Verification items for the finished model (mm, model axes). Face numbers are marked on the shaded views. A direction names the side the tool comes from. Give positions to 0.01 mm unless a question says otherwise; leave off trailing zeros. Loops run counter-clockwise (first coordinate to the right, second up) from the corner with the lowest first, then second, coordinate; pieces in that order, holes last. Notation, with made-up numbers: M 36.5,14.5 L 91.5,14.5 A33 ccw 91.5,46.5 Z; hole C -39,10 d4. An arc over 180 degrees is marked long. Answer in a Markdown table with one row per item.
```python
from build123d import *

# Parameters (mm, degrees)
ESBO_O1_W                        = 56
ESBO_O1_H                        = 28.051471863
RESSALTO_EXTRUS_O1_DEPTH         = 16
CORTE_EXTRUS_O1_DEPTH            = 100
ESBO_O3_W                        = 18
ESBO_O3_H                        = 28.051471863
CORTE_EXTRUS_O2_DEPTH            = 5
FURO_COM_FOLGA_DE_M32_D          = 3.4
FURO_COM_FOLGA_DE_M34_D          = 3.4
CHANFRO1_SIZE                    = 5
CORTE_EXTRUS_O3_DEPTH            = 8
RESSALTO_EXTRUS_O3_DEPTH         = 56
CORTE_EXTRUS_O4_DEPTH            = 100
CHANFRO2_START                   = 38.631741411
CHANFRO2_OUTLINE_W               = 9
CHANFRO2_OUTLINE_H               = 10
CHANFRO2_DEPTH                   = 4.368258589
CHANFRO3_START                   = -67
CHANFRO3_OUTLINE_W               = 9
CHANFRO3_OUTLINE_H               = 10
CHANFRO3_DEPTH                   = 3.439248526
RESSALTO_EXTRUS_O4_DEPTH         = 2
CORTE_EXTRUS_O5_DEPTH            = 100
CORTE_EXTRUS_O6_START            = -56
ESBO_O24_W                       = 1.5
ESBO_O24_H                       = 30.126471863
CORTE_EXTRUS_O6_DEPTH            = 56
RESSALTO_EXTRUS_O6_DEPTH         = 17
RESSALTO_EXTRUS_O7_START         = -17
RESSALTO_EXTRUS_O7_DEPTH         = 17
ESBO_O29_R                       = 1.7
CORTE_EXTRUS_O16_DEPTH           = 17
CORTE_EXTRUS_O16_DRAFT           = -0.2
CORTE_EXTRUS_O16_PROFILE_2_DEPTH = 17
CORTE_EXTRUS_O16_PROFILE_2_DRAFT = -0.2


with BuildPart() as part:
    # Esboço1 → Ressalto-extrusão1 (new body)
    with BuildSketch(Plane.XY):
        with Locations((-21.244121058, 34.04115584)):
            Rectangle(ESBO_O1_W, ESBO_O1_H)
    extrude(amount=RESSALTO_EXTRUS_O1_DEPTH)

    # Esboço2 → Corte-extrusão1 (cut)
    with BuildSketch(Plane(origin=(6.755878942, 0, 0), x_dir=(0, 0, -1), z_dir=(1, 0, 0))):
        with BuildLine():
            Line((0, 41.428078682), (0, 30.602761135))
            ThreePointArc((0, 30.602761135), (-6.875, 27.265419908), (-13.75, 30.602761135))
            Line((-13.75, 30.602761135), (-13.75, 41.428078682))
            ThreePointArc((-13.75, 41.428078682), (-6.875, 44.765419908), (0, 41.428078682))
        make_face()
    extrude(amount=-CORTE_EXTRUS_O1_DEPTH, mode=Mode.SUBTRACT)

    # Esboço3 → Corte-extrusão2 (cut)
    with BuildSketch(Plane.XY.offset(16)):
        with Locations((-21.244121058, 34.04115584)):
            Rectangle(ESBO_O3_W, ESBO_O3_H)
    extrude(amount=-CORTE_EXTRUS_O2_DEPTH, mode=Mode.SUBTRACT)

    # Furo com folga de M32 (through all)
    with Locations(Plane.XY.offset(16)):
        with Locations((-1.994121058, 45.566891771), (-40.494121058, 45.566891771)):
            Hole(FURO_COM_FOLGA_DE_M32_D / 2)

    # Furo com folga de M34 (through all)
    with Locations(Plane.XY.offset(16)):
        with Locations((-1.994121058, 24.015419908), (-40.494121058, 24.015419908)):
            Hole(FURO_COM_FOLGA_DE_M34_D / 2)

    # Chanfro1
    # the kernel refuses this chamfer: 5 mm, written as the material it takes off along each edge
    with BuildSketch(Plane(origin=(-12.244121058, 7.157004969, 16), x_dir=(1, 0, 0), z_dir=(0, 1, 0))) as chanfro1_piece_1:
        Polygon((CHANFRO1_SIZE, 0), (0, CHANFRO1_SIZE), (0, 0), align=None)
    extrude(amount=53.768301742, mode=Mode.SUBTRACT)
    with BuildSketch(Plane(origin=(-30.244121058, 60.925306711, 16), x_dir=(0, 0, -1), z_dir=(0, -1, 0))) as chanfro1_piece_2:
        Polygon((CHANFRO1_SIZE, 0), (0, -CHANFRO1_SIZE), (0, 0), align=None)
    extrude(amount=53.768301742, mode=Mode.SUBTRACT)

    # Esboço17 → Corte-extrusão3 (cut)
    with BuildSketch(Plane.XY.offset(11)):
        with BuildLine():
            Line((-20.044121058, 25.869616944), (-22.444121058, 25.869616944))
            ThreePointArc((-22.444121058, 25.869616944), (-23.151227839, 26.162510163), (-23.444121058, 26.869616944))
            Line((-23.444121058, 26.869616944), (-23.444121058, 27.069616944))
            Line((-23.444121058, 27.069616944), (-23.444121058, 44.959616944))
            Line((-23.444121058, 44.959616944), (-23.444121058, 45.159616944))
            ThreePointArc((-23.444121058, 45.159616944), (-23.151227839, 45.866723726), (-22.444121058, 46.159616944))
            Line((-22.444121058, 46.159616944), (-20.044121058, 46.159616944))
            ThreePointArc((-20.044121058, 46.159616944), (-19.337014277, 45.866723726), (-19.044121058, 45.159616944))
            Line((-19.044121058, 45.159616944), (-19.044121058, 43.159616944))
            Line((-19.044121058, 43.159616944), (-19.044121058, 36.014616944))
            Line((-19.044121058, 36.014616944), (-19.044121058, 26.869616944))
            ThreePointArc((-19.044121058, 26.869616944), (-19.337014277, 26.162510163), (-20.044121058, 25.869616944))
        make_face()
    extrude(amount=-CORTE_EXTRUS_O3_DEPTH, mode=Mode.SUBTRACT)

    # Esboço20 → Ressalto-extrusão3 (add)
    with BuildSketch(Plane.ZY.offset(49.244121058)):
        Polygon((0, 48.066891771), (16, 48.066891771), (16, 48.866891771), align=None)
    extrude(amount=-RESSALTO_EXTRUS_O3_DEPTH)

    # Esboço21 → Corte-extrusão4 (cut)
    with BuildSketch(Plane.XZ.offset(-48.066891771)):
        Polygon((-7.244121058, 16), (-12.244121058, 11), (-30.244121058, 11), (-35.244121058, 16), align=None)
    extrude(amount=-CORTE_EXTRUS_O4_DEPTH, mode=Mode.SUBTRACT)

    # Chanfro2: read off the stored shape, not the designer's step
    # Chanfro2 outline → Chanfro2 (cut)
    with BuildSketch(Plane(origin=(0, 0, 0), x_dir=(0.8097846116702572, -0.42511166270745215, -0.4043871374464777), z_dir=(0.586727264324789, 0.58672726432479, 0.558123852380363)).offset(CHANFRO2_START)):
        with Locations((-22.5, 22)):
            Rectangle(CHANFRO2_OUTLINE_W, CHANFRO2_OUTLINE_H)
    extrude(amount=CHANFRO2_DEPTH, mode=Mode.SUBTRACT)

    # Chanfro3: read off the stored shape, not the designer's step
    # Chanfro3 outline → Chanfro3 (cut)
    with BuildSketch(Plane(origin=(0, 0, 0), x_dir=(0.8097846116702566, 0.4251116627074525, 0.404387137446478), z_dir=(0.5867272643247896, -0.5867272643247896, -0.5581238523803627)).offset(CHANFRO3_START)):
        with Locations((-11.5, -22)):
            Rectangle(CHANFRO3_OUTLINE_W, CHANFRO3_OUTLINE_H)
    extrude(amount=CHANFRO3_DEPTH, mode=Mode.SUBTRACT)

    # Esboço22 → Ressalto-extrusão4 (add)
    with BuildSketch(Plane.XZ.offset(-20.015419908)):
        Polygon((-49.244121058, 16), (-35.244121058, 16), (-30.244121058, 11), (-12.244121058, 11), (-7.244121058, 16), (6.755878942, 16), (6.755878942, 0), (-49.244121058, 0), align=None)
    extrude(amount=RESSALTO_EXTRUS_O4_DEPTH)

    # Esboço23 → Corte-extrusão5 (cut)
    with BuildSketch(Plane.ZY.offset(49.244121058)):
        Polygon((0, 18.015419908), (16, 19.091373139), (16, 18.015419908), align=None)
    extrude(amount=-CORTE_EXTRUS_O5_DEPTH, mode=Mode.SUBTRACT)

    # Esboço24 → Corte-extrusão6 (cut)
    with BuildSketch(Plane(origin=(6.755878942, 0, 0), x_dir=(0, 0, -1), z_dir=(1, 0, 0)).offset(CORTE_EXTRUS_O6_START)):
        with Locations((-0.75, 33.07865584)):
            Rectangle(ESBO_O24_W, ESBO_O24_H)
    extrude(amount=CORTE_EXTRUS_O6_DEPTH, mode=Mode.SUBTRACT)

    # Esboço26 → Ressalto-extrusão6 (add)
    with BuildSketch(Plane(origin=(6.755878942, 0, 0), x_dir=(0, 0, -1), z_dir=(1, 0, 0))):
        with BuildLine():
            ThreePointArc((-13.75, 41.428078682), (-7.807709843, 43.777058017), (-1.47808403, 42.902785008))
            ThreePointArc((-1.47808403, 42.902785008), (-7.918969725, 44.702918237), (-13.75, 41.428078682))
        make_face()
    extrude(amount=-RESSALTO_EXTRUS_O6_DEPTH)

    # Esboço28 → Ressalto-extrusão7 (add)
    with BuildSketch(Plane.ZY.offset(49.244121058).offset(RESSALTO_EXTRUS_O7_START)):
        with BuildLine():
            ThreePointArc((13.75, 41.428078682), (7.932773281, 44.701248348), (1.5, 42.919902148))
            ThreePointArc((1.5, 42.919902148), (7.808321968, 43.679325435), (13.75, 41.428078682))
        make_face()
    extrude(amount=RESSALTO_EXTRUS_O7_DEPTH)


with BuildPart() as corte_extrus_o16_tool:
    # Esboço29 → Corte-extrusão16 (with draft: the straight prism first)
    with BuildSketch(Plane.XY.offset(16)):
        with Locations((-40.494121058, 45.566891771)):
            Circle(ESBO_O29_R)
    extrude(amount=-CORTE_EXTRUS_O16_DEPTH)
    # Corte-extrusão16: the draft: its side faces are tilted about the plane it starts from
    corte_extrus_o16_sides = [corte_extrus_o16_tool.faces().sort_by_distance(p)[0] for p in [
        (-42.194121058, 45.566891771, 7.5),
    ]]
    draft(corte_extrus_o16_sides, Plane.XY.offset(16), CORTE_EXTRUS_O16_DRAFT)


with BuildPart() as part_1:
    add(part.part)

    # Corte-extrusão16: cut by corte_extrus_o16_tool
    add(corte_extrus_o16_tool.part, mode=Mode.SUBTRACT)


with BuildPart() as corte_extrus_o16_profile_2_tool:
    # Esboço29 → Corte-extrusão16 profile 2 (with draft: the straight prism first)
    with BuildSketch(Plane.XY.offset(16)):
        with Locations((-1.994121058, 45.566891771)):
            Circle(ESBO_O29_R)
    extrude(amount=-CORTE_EXTRUS_O16_PROFILE_2_DEPTH)
    # Corte-extrusão16 profile 2: the draft: its side faces are tilted about the plane it starts from
    corte_extrus_o16_profile_2_sides = [corte_extrus_o16_profile_2_tool.faces().sort_by_distance(p)[0] for p in [
        (-3.694121058, 45.566891771, 7.5),
    ]]
    draft(corte_extrus_o16_profile_2_sides, Plane.XY.offset(16), CORTE_EXTRUS_O16_PROFILE_2_DRAFT)


with BuildPart() as part_2:
    add(part_1.part)

    # Corte-extrusão16 profile 2: cut by corte_extrus_o16_profile_2_tool
    add(corte_extrus_o16_profile_2_tool.part, mode=Mode.SUBTRACT)


solid = part_2.part
```
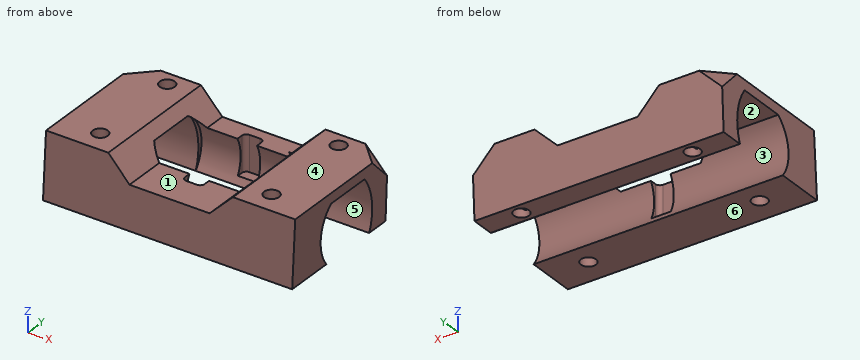
Item 1: Scan lines: L1, parallel to Y at x = -1, z = 9.5; L2, parallel to X at y = 46, z = 6.75; L3, parallel to Z at x = -25.5, y = 20. Record each from-to range of solid material in increasing order. Write a range as [from, to].
Reported:
| item | result |
|---|---|
| L1 | y = [18.65, 22.64], [25.39, 27.67], [43.45, 44.22], [46.95, 48.54] |
| L2 | x = [-49.24, -42.14], [-38.85, -22.99], [-19.5, -3.64], [-0.35, 6.76] |
| L3 | z = [1.5, 11] |
Item 2: Sectioned sample at A-A (z = 6). State how many separate pieces and enclosed holes the cut face has, and give its area (3 significant figures).
Reported:
| item | result |
|---|---|
| separate pieces | 2 |
| enclosed holes | 4 |
| area | 685 mm^2 |
Item 3: Tool access check on the marked faces 1, 2 and 3. Record the directions out of +Z, -Z, +X, -X, +Y, -Y that give a thin tool (end or side, any length) a straight path to the whole face; none if there is none.
Reported:
| item | result |
|---|---|
| face 1 | +Z, +Y, -Y |
| face 2 | -Z, +X, -X |
| face 3 | +X, -X |
Item 4: Sectioned sample at C-C (y = 38). Record the cut outline in (x, z), and give its area (3 significant figures).
Reported:
| item | result |
|---|---|
| outline | M -49.24,13.75 L -32.99,13.75 L -35.24,16 L -49.24,16 Z; M -9.49,13.75 L 6.76,13.75 L 6.76,16 L -7.24,16 Z |
| area | 68.1 mm^2 |
Item 5: Sectioned sample at B-B (x = -26). Record the cut outline in (y, z) (3 decimals), and give its area (3 significant figures).
Reported:
| item | result |
|---|---|
| outline | M 18.116,1.5 L 29.111,1.5 A8.75 cw 28.299,11 L 18.755,11 Z; M 42.92,1.5 L 48.142,1.5 L 48.617,11 L 43.732,11 A8.75 cw Z |
| area | 127 mm^2 |
Item 6: Release check for a two-part mould opening along Z. For the marked faces 4, 5 and 6 record: released by +Z, released by -Z, zero draft, split by the parting line, or undercut.
Reported:
| item | result |
|---|---|
| face 4 | released by +Z |
| face 5 | undercut |
| face 6 | released by -Z |
Item 7: Sectioned sample at D-D (y = 21.5). Record the cut outline in (x, z).
Reported:
| item | result |
|---|---|
| outline | M -49.24,1.5 L 6.76,1.5 L 6.76,16 L -7.24,16 L -12.24,11 L -30.24,11 L -35.24,16 L -49.24,16 Z |
Item 8: Go/stop test with flat-tipped pins: pin 1 (4 mm diameter, centred on x = -19.5, y = 26.5, fed in from +Z); pin 2 (0.7 mm diameter, centred on x = -21, z = 6, fed in from +Y); pin 3 (5 mm diameter, centred on x = 0.5, z = 10.5, fed in from -Y); pin 4 (2.5 mm diameter, centred on x = -1.99, y = 45.57, fed in from -Z). Record where each tip stops, or that it passes through.
Reported:
| item | result |
|---|---|
| pin 1 | stops at z = 11 |
| pin 2 | stops at y = 48.38 |
| pin 3 | stops at y = 18.55 |
| pin 4 | passes through |
